Build history of the part. All positions in model axes, mm. A direction names the side the tool comes from. Give positions to 0.01 mm unless a question says otherwise; leave off trailing zeros. Loops run counter-clockwise (first coordinate to the right, second up) from the corner with the lowest first, then second, coordinate; pieces in that order, holes last. Notation, with made-up numbers: (79.25, 53) - (99.25, 53) arc R9 cw to (99.25, 66) - close; hole circle Ø5 at (32, 28.5). An arc over 180 degrees is marked (long way). Return JSON: item names as keys, results as strings. Group by question number.
1) Mould opens along Z. For faces 4 (the face through (2.6, 2, -4.5)), 5 (the face through (-1, -9, 4)), 6 (the face through (0, 0, -6)), 7 (the face through (3, -0.1, -0.5)) say: released by +Z, released by -Z, zero draft, split by the parting line, or undercut.
2) Slice it at A-A (z = -3.25). List the corners of the cut face in (x, y).
3) Slice it at D-D (z = 3.5). List the corners of the cut face in (x, y).
4) Slice it at C-C (y = -9.75). List the corners of the cut face in (x, z), and give its area (3 significant figures).
5) 3-axis set-ups, long thin cutter, end or side, ignore diameter. For faces 1 (the face through (-0.488, -10.521, 1.304)), 2 (the face through (-2.6, 2, -4.5)), 3 (the face through (3, -2.5, -4.7)): which of +Z, -Z, +X, -X, +Y, -Y reach the whole face in a straight line?
6) Drop flat-ended pins along their axis: pin 1 (5 mm diameter, centred on y = -8.5, z = 3.5, fed in from +X); pin 2 (0.6 mm diameter, centred on x = 0, z = 3.5, fed in from -Y); pin 3 (0.8 mm diameter, centred on x = 2.5, z = -4.5, fed in from -Y). Give the stop position or say it passes through.
7) Drill centre lines: probe 1 along Z at (x, y) = (0, -10); probe 2 along Z at (x, y) = (0, -8.15); probe 3 along Y at (x, z) = (-3, 0.5). Where is each one in solid material? Low to high. Write a range as from..to.
8) Slice it at B-B (x = 0). List the corners of the cut face in (y, z).
Autodesk Inventor part; units mm, degrees
ref_plane "YZ Plane" through (0, 0, 0) normal (1, 0, 0) x (0, 1, 0)
ref_plane "XZ Plane" through (0, 0, 0) normal (0, 1, 0) x (-1, 0, 0)
ref_plane "XY Plane" through (0, 0, 0) normal (0, 0, 1) x (1, 0, 0)
sketch "Skizze1" plane through (0, 0, 0) normal (0, 0, 1) x (1, 0, 0)
  line L0 (-3.5, -3.5) -> (3.5, -3.5)
  line L1 (3.5, -3.5) -> (3.5, 3.5)
  line L2 (3.5, 3.5) -> (-3.5, 3.5)
  line L3 (-3.5, 3.5) -> (-3.5, -3.5)
  line L4 (-3.5, -3.5) -> (3.5, 3.5) construction
  line L5 (3.5, -3.5) -> (-3.5, 3.5) construction
  point P0 (0, 0)
  dimension "d0" = 7
  dimension "d1" = 7
extrude "Extrusion1" add sketch "Skizze1" along normal blind 7
sketch "Skizze2" plane through (0, 0, 0) normal (0, 0, -1) x (-1, 0, 0)
  circle A0 centre (0, 0) radius 3
  dimension "d4" = 6
extrude "Extrusion2" add sketch "Skizze2" along normal blind 1
sketch "Skizze3" plane through (0, 0, -1) normal (0, 0, -1) x (-1, 0, 0)
  line L0 (3.5, 3.5) -> (-3.5, 3.5)
  line L1 (-3.5, 3.5) -> (-3.5, -3.5)
  line L2 (-3.5, -3.5) -> (3.5, -3.5)
  line L3 (3.5, -3.5) -> (3.5, 3.5)
  line L4 (3.5, 3.5) -> (-3.5, -3.5) construction
  line L5 (-3.5, 3.5) -> (3.5, -3.5) construction
  point P0 (0, 0)
  dimension "d7" = 7
  dimension "d8" = 7
extrude "Extrusion3" add sketch "Skizze3" along normal blind 1.5
sketch "Skizze4" plane through (0, 0, -2.5) normal (0, 0, -1) x (-1, 0, 0)
  line L0 (3.5, 3.5) -> (-3.5, 3.5)
  line L1 (-3.5, 3.5) -> (-3.5, -3.5)
  line L2 (-3.5, -3.5) -> (3.5, -3.5)
  line L3 (3.5, -3.5) -> (3.5, 3.5)
  line L4 (-3.5, 3.5) -> (3.5, 3.5)
  line L5 (3.5, 3.5) -> (2, 3.5)
  line L6 (2, 3.5) -> (2, 2)
  line L7 (2, 2) -> (3.5, 2)
  line L8 (3.5, 2) -> (3.5, 3.5)
  line L9 (3.5, -3.5) -> (-3.5, -3.5)
  line L10 (3.5, -3.5) -> (2, -3.5)
  line L11 (2, -3.5) -> (2, -2)
  line L12 (2, -2) -> (3.5, -2)
  line L13 (3.5, -2) -> (3.5, -3.5)
  line L14 (-3.5, 3.5) -> (-2, 3.5)
  line L15 (-2, 3.5) -> (-2, 2)
  line L16 (-2, 2) -> (-3.5, 2)
  line L17 (-3.5, 2) -> (-3.5, 3.5)
  line L18 (-3.5, -3.5) -> (-3.5, 3.5)
  line L19 (-3.5, -3.5) -> (-2, -3.5)
  line L20 (-2, -3.5) -> (-2, -2)
  line L21 (-2, -2) -> (-3.5, -2)
  line L22 (-3.5, -2) -> (-3.5, -3.5)
  point P0 (0, 0)
  dimension "d11" = 1.5
  dimension "d12" = 1.5
  dimension "d13" = 1.5
  dimension "d14" = 1.5
  dimension "d15" = 1.5
  dimension "d16" = 1.5
  dimension "d17" = 1.5
  dimension "d18" = 1.5
extrude "Extrusion4" add sketch "Skizze4" along normal blind 0.5 contours L3 L7 L6 L0 | L15 L16 L1 L0 | L3 L2 L11 L12 | L21 L20 L2 L1
sketch "Skizze5" plane through (0, 0, -3) normal (0, 0, -1) x (-1, 0, 0)
  line L0 (3.5, -3.5) -> (3.5, -2)
  line L1 (3.5, -2) -> (2, -2)
  line L2 (2, -2) -> (2, -3.5)
  line L3 (2, -3.5) -> (3.5, -3.5)
  line L4 (-3.5, -3.5) -> (-2, -3.5)
  line L5 (-2, -3.5) -> (-2, -2)
  line L6 (-2, -2) -> (-3.5, -2)
  line L7 (-3.5, -2) -> (-3.5, -3.5)
  line L8 (-3.5, 3.5) -> (-3.5, 2)
  line L9 (-3.5, 2) -> (-2, 2)
  line L10 (-2, 2) -> (-2, 3.5)
  line L11 (-2, 3.5) -> (-3.5, 3.5)
  line L12 (3.5, 3.5) -> (2, 3.5)
  line L13 (2, 3.5) -> (2, 2)
  line L14 (2, 2) -> (3.5, 2)
  line L15 (3.5, 2) -> (3.5, 3.5)
  line L16 (2, -2) -> (3, -2)
  line L17 (3, -2) -> (3, -3)
  line L18 (3, -3) -> (2, -3)
  line L19 (2, -3) -> (2, -2)
  line L20 (-2, -2) -> (-3, -2)
  line L21 (-3, -2) -> (-3, -3)
  line L22 (-3, -3) -> (-2, -3)
  line L23 (-2, -3) -> (-2, -2)
  line L24 (-2, 2) -> (-3, 2)
  line L25 (-3, 2) -> (-3, 3)
  line L26 (-3, 3) -> (-2, 3)
  line L27 (-2, 3) -> (-2, 2)
  line L28 (2, 2) -> (3, 2)
  line L29 (3, 2) -> (3, 3)
  line L30 (3, 3) -> (2, 3)
  line L31 (2, 3) -> (2, 2)
  point P0 (0, 0)
  dimension "d21" = 1
  dimension "d22" = 1
  dimension "d23" = 1
  dimension "d24" = 1
  dimension "d25" = 1
  dimension "d26" = 1
  dimension "d27" = 1
  dimension "d28" = 1
extrude "Extrusion5" add sketch "Skizze5" along normal blind 3.5 contours L17 L18 L2 L1 | L22 L21 L6 L5 | L25 L26 L10 L9 | L30 L29 L14 L13
sketch "Skizze6" plane through (0, 0, -2.5) normal (0, 0, -1) x (-1, 0, 0)
  circle A0 centre (0, 0) radius 0.5
  dimension "d31" = 1
extrude "Extrusion6" add sketch "Skizze6" along normal blind 3.5
sketch "Skizze7" plane through (-3.5, -3.5, 0) normal (0, -1, 0) x (1, 0, 0)
  line L0 (0, 0) -> (7, 0)
  line L1 (7, 0) -> (7, 7)
  line L2 (0, 7) -> (7, 7)
  line L3 (0, 0) -> (0, 7)
  line L4 (0, 0) -> (0, 7) construction
  line L5 (0, 3.5) -> (7, 3.5) construction
  line L6 (3.5, 7) -> (3.5, 0) construction
  circle A0 centre (3.5, 3.5) radius 2.75
  dimension "d34" = 5.5
extrude "Extrusion7" add sketch "Skizze7" along normal blind 8.5 contours A0
thread "Gewinde1"
sketch "Skizze8" plane through (0, -12, 3.5) normal (0, -1, 0) x (1, 0, 0)
  circle A0 centre (0, 0) radius 2.75
  circle A1 centre (0, 0) radius 2.25
  point P0 (0, -3.5)
  dimension "d39" = 4.5
extrude "Extrusion8" cut sketch "Skizze8" against normal blind 3 contours A1
sketch "Skizze9" plane through (0, -9, 3.5) normal (0, -1, 0) x (1, 0, 0)
  circle A0 centre (0, 0) radius 2.25
  circle A1 centre (0, 0) radius 0.4
  point P0 (0, -3.5)
  dimension "d42" = 0.8
extrude "Extrusion9" cut sketch "Skizze9" against normal blind 3 contours A1
properties part number "SMA-F-RA" material "Messing, weicher Gelbton"
Results:
{
 "1": {"face 4": "zero draft", "face 5": "undercut", "face 6": "released by -Z", "face 7": "undercut"},
 "2": {"outline": "(-3, -3) - (-2, -3) - (-2, -2) - (-3, -2) - close; (-3, 2) - (-2, 2) - (-2, 3) - (-3, 3) - close; circle Ø1 at (0, 0); (2, -3) - (3, -3) - (3, -2) - (2, -2) - close; (2, 2) - (3, 2) - (3, 3) - (2, 3) - close"},
 "3": {"outline": "(-3.5, -3.5) - (-2.75, -3.5) - (-2.75, -12) - (-2.25, -12) - (-2.25, -9) - (-0.4, -9) - (-0.4, -6) - (0.4, -6) - (0.4, -9) - (2.25, -9) - (2.25, -12) - (2.75, -12) - (2.75, -3.5) - (3.5, -3.5) - (3.5, 3.5) - (-3.5, 3.5) - close"},
 "4": {"outline": "circle Ø5.5 at (0, 3.5); hole circle Ø4.5 at (0, 3.5)", "area": "7.85 mm2"},
 "5": {"face 1": "-Y", "face 2": "-Z, +X, -X", "face 3": "-Z, +X, +Y, -Y"},
 "6": {"pin 1": "x = 2.75", "pin 2": "y = -6", "pin 3": "y = -3"},
 "7": {"probe 1": "0.75..1.25, 5.75..6.25", "probe 2": "0.75..3.1, 3.9..6.25", "probe 3": "-3.5..3.5"},
 "8": {"outline": "(-12, 0.75) - (-3.5, 0.75) - (-3.5, 0) - (-3, 0) - (-3, -1) - (-3.5, -1) - (-3.5, -2.5) - (-0.5, -2.5) - (-0.5, -6) - (0.5, -6) - (0.5, -2.5) - (3.5, -2.5) - (3.5, -1) - (3, -1) - (3, 0) - (3.5, 0) - (3.5, 7) - (-3.5, 7) - (-3.5, 6.25) - (-12, 6.25) - (-12, 5.75) - (-9, 5.75) - (-9, 3.9) - (-6, 3.9) - (-6, 3.1) - (-9, 3.1) - (-9, 1.25) - (-12, 1.25) - close"}
}
